Source: CAD feature listing. Evaluate the final solid. Frame: model axes, mm. Face numbers are marked on the shaded views. Give positions to 0.01 mm unless a question says otherwise; leave off trailing zeros. Loops run counter-clockwise (first coordinate to the right, second up) from the corner with the lowest first, then second, coordinate; pieces in that order, holes last. Notation, with made-up numbers: (-8, 70) -> (49, 70) arc R13 cw to (49, 92) -> close; hole circle Ø9 at (70, 24). An arc over 180 degrees is marked (long way). Put each result on its own line as item: value.
```python
from build123d import *

# Parameters (mm, degrees)
F0_R     = 28.575
F1_DEPTH = 19.05
F2_R     = 4.7625
F3_DEPTH = 9.525
F4_R     = 4.7625
F5_DEPTH = 9.525


with BuildPart() as f1:
    # F0 (on Top) → F1 (new body)
    with BuildSketch(Plane.XY):
        Circle(F0_R)
    extrude(amount=F1_DEPTH)

    # F2 (on Top) → F3 (join)
    with BuildSketch(Plane.XY):
        Circle(F2_R)
    extrude(amount=F3_DEPTH)

    # F4 (on face) → F5 (cut)
    with BuildSketch(Plane(origin=(0, 0, 0), x_dir=(1, 0, 0), z_dir=(0, 0, -1))):
        Circle(F4_R)
    extrude(amount=-F5_DEPTH, mode=Mode.SUBTRACT)


solid = f1.part
```
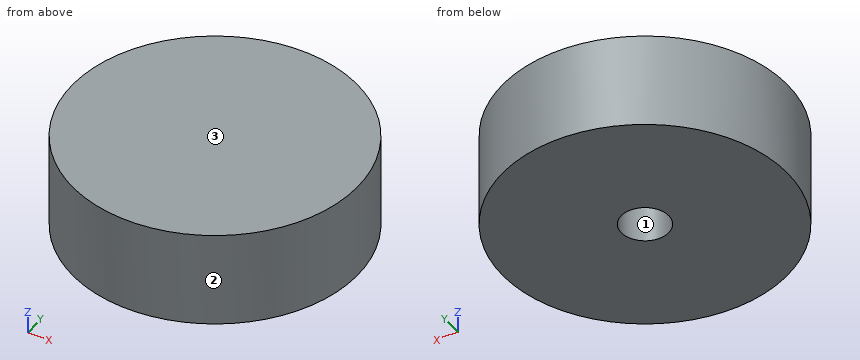
(1) First-contact query: P1, Ø5, axis at x = 1.5, z = 6, coming from the -Y side (3 decimals); P2, Ø10, axis at x = 11, z = 16, coming from the +Y side; P3, Ø1.5, axis at x = -18.5, z = 3.5, coming from the -Y side. Flat tips, straight axial feed; report the tip coordinate or a pass-through.
Calculated:
P1: stops at y = -28.575
P2: stops at y = 27.94
P3: stops at y = -22.39
(2) Section D-D on z = 17.5. Return loops of the section in (x, y) (3 decimals).
Calculated:
outline: circle Ø57.15 at (0, 0)
(3) Draft query along X for the marked faces 1, 2 and 3. Return one class per face: released by +X, released by -X, zero draft, split by the parting line, or undercut.
Calculated:
face 1: undercut
face 2: split by the parting line
face 3: zero draft
(4) Line query: probe 1 along Y at (x, z) = (0, 7.25) (1 decimal); probe 2 along Y at (x, z) = (-0.5, 16.5); probe 3 along X at (y, z) = (3, 8.75). Output: solid intervals per line, ascending. Write a range as from..to.
Calculated:
probe 1: y = -28.6..-4.8, 4.8..28.6
probe 2: y = -28.57..28.57
probe 3: x = -28.42..-3.7, 3.7..28.42
